from build123d import *

# Parameters (mm, degrees)
SKETCH1_W           = 2133.6
SKETCH1_H           = 762
BOSS_EXTRUDE1_DEPTH = 50.8
SKETCH3_W           = 114.3
SKETCH3_H           = 279.4
BOSS_EXTRUDE2_DEPTH = 508
SKETCH4_W           = 2133.6
SKETCH4_H           = 279.4
BOSS_EXTRUDE3_DEPTH = 50.8
SKETCH5_W           = 2133.6
SKETCH5_H           = 50.8
BOSS_EXTRUDE4_DEPTH = 127


with BuildPart() as part:
    # Sketch1 → Boss-Extrude1 (new body)
    with BuildSketch(Plane(origin=(0, 0, 0), x_dir=(1, 0, 0), z_dir=(0, 1, 0))):
        Rectangle(SKETCH1_W, SKETCH1_H)
    extrude(amount=BOSS_EXTRUDE1_DEPTH)

    # Sketch3 → Boss-Extrude2 (add)
    with BuildSketch(Plane(origin=(0, 50.8, 0), x_dir=(1, 0, 0), z_dir=(0, 1, 0))):
        with Locations((-1009.65, 241.3)):
            Rectangle(SKETCH3_W, SKETCH3_H)
        with Locations((1009.65, 241.3)):
            Rectangle(SKETCH3_W, SKETCH3_H)
    extrude(amount=BOSS_EXTRUDE2_DEPTH)

    # Sketch4 → Boss-Extrude3 (add)
    with BuildSketch(Plane(origin=(0, 558.8, 0), x_dir=(1, 0, 0), z_dir=(0, 1, 0))):
        with Locations((0, 241.3)):
            Rectangle(SKETCH4_W, SKETCH4_H)
    extrude(amount=BOSS_EXTRUDE3_DEPTH)

    # Sketch5 → Boss-Extrude4 (add)
    with BuildSketch(Plane.XY.offset(-101.6)):
        with Locations((0, 584.2)):
            Rectangle(SKETCH5_W, SKETCH5_H)
    extrude(amount=BOSS_EXTRUDE4_DEPTH)


solid = part.part
Read the model definition and answer for the solid it produces. Units are mm, in the model's axes. A direction names the side the tool comes from. Coordinates: 2 decimals unless noted, no trailing zeros. Order: outer loops, then holes, each group sorted by start corner. A loop starts at its lowest first (then second) coordinate and runs counter-clockwise, first axis right, second up. Notation, with made-up numbers: (55.5, -30) - (66.5, -30) arc R28 cw to (66.5, -11) - close; hole circle Ø2 at (-34, 70.5). An arc over 180 degrees is marked (long way). Use one line per item in the form item = value.
(1) For a pull along X with two mould halves and no side action, classify faces 4 (the face through (-15, 0, -5)), 5 (the face through (-952.5, 301, -239)), 6 (the face through (-1066.8, 301, -175)) as pulls with the +X half, pulls with the -X half, needs draft (parallel to the pull), parting line crosses it, or undercut.
Computed values:
face_4 = needs draft
face_5 = undercut
face_6 = pulls with the -X half
(2) Section B-B, the plane y = 86.5 is taken. Give the vertices of the cut face in (x, z), then the cut area to 3 significant figures.
Computed values:
outline = (-1066.8, -381) - (-952.5, -381) - (-952.5, -101.6) - (-1066.8, -101.6) - close; (952.5, -381) - (1066.8, -381) - (1066.8, -101.6) - (952.5, -101.6) - close
area = 63,900 mm²
(3) Given pin 1 Ø15 at (x, y) = (219, 580) entering from +Z; pin 2 Ø2 at (x, z) = (-774.5, 253.5) entering from -Y, each flat-ended and moving along its own axis, determine where each tip first touches the part or whether it passes through.
Computed values:
pin_1 = 25.4
pin_2 = 0
(4) Section A-A, the plane z = -18.5 is taken. Give the vertices of the cut face in (x, y), then the cut area to 3 significant figures.
Computed values:
outline = (-1066.8, 0) - (1066.8, 0) - (1066.8, 50.8) - (-1066.8, 50.8) - close; (-1066.8, 558.8) - (1066.8, 558.8) - (1066.8, 609.6) - (-1066.8, 609.6) - close
area = 217,000 mm²
(5) Section C-C, the plane z = 74.5 is taken. Give the vertices of the cut face in (x, y).
Computed values:
outline = (-1066.8, 0) - (1066.8, 0) - (1066.8, 50.8) - (-1066.8, 50.8) - close
(6) Straight lines are drawn through the part: L1, parallel to X at y = 351.5, z = -282; L2, parallel to Y at x = -965, z = 24; L3, parallel to Y at x = 617, z = 51.5. For each, find the intervals that lie inside material, in ascending order.
Computed values:
L1 = -1066.8 to -952.5, 952.5 to 1066.8
L2 = 0 to 50.8, 558.8 to 609.6
L3 = 0 to 50.8
(7) Which of the six approach directions +Z, -Z, +X, -X, +Y, -Y give full straight-line access (tool end or side, diameter ignored) to faces 1 (the face through (1009, 301, -101.6)), 2 (the face through (-15, 585, 25.4)), 3 (the face through (952.5, 301, -239))?
Computed values:
face_1 = +Z, +X, -X
face_2 = +Z, +X, -X, +Y
face_3 = +Z, -Z
